from build123d import *

# Parameters (mm, degrees)
SKETCH1_W               = 202.2
SKETCH1_H               = 40
SKETCH1_R               = 1.65
BOSS_EXTRUDE1_DEPTH     = 4
SKETCH2_W               = 162.2
SKETCH2_H               = 40
CUT_EXTRUDE1_DEPTH      = 4
BOSS_EXTRUDE3_DEPTH     = 40
CUT_EXTRUDE2_DEPTH      = 184.624181414
CUT_EXTRUDE2_DEPTH_BACK = 184.624181414
SKETCH4_R               = 1.5
CUT_EXTRUDE3_DEPTH      = 104.644633243
CUT_EXTRUDE3_DEPTH_BACK = 104.644633243
SKETCH5_R               = 1.5


with BuildPart() as part:
    # Sketch1 → Boss-Extrude1 (new body)
    with BuildSketch(Plane.XY):
        Rectangle(SKETCH1_W, SKETCH1_H)
        with Locations((-95.1, 10)):
            Circle(SKETCH1_R, mode=Mode.SUBTRACT)
        with Locations((-95.1, -10)):
            Circle(SKETCH1_R, mode=Mode.SUBTRACT)
        with Locations(Location((95.1, -10, 0), (0, 0, 180))):
            Circle(SKETCH1_R, mode=Mode.SUBTRACT)
        with Locations(Location((95.1, 10, 0), (0, 0, 180))):
            Circle(SKETCH1_R, mode=Mode.SUBTRACT)
    extrude(amount=BOSS_EXTRUDE1_DEPTH)

    # Sketch2 → Cut-Extrude1 (cut)
    with BuildSketch(Plane.XY.offset(4)):
        Rectangle(SKETCH2_W, SKETCH2_H)
    extrude(amount=-CUT_EXTRUDE1_DEPTH, mode=Mode.SUBTRACT)


with BuildPart() as cut_extrude1_piece_1:
    # of the separate pieces the step leaves, piece 1, a body of its own (cut_extrude1_pieces)
    add(part.part.solids().sort_by_distance((-101.1, 20, 0))[0])



with BuildPart() as cut_extrude1_piece_2:
    # of the separate pieces the step leaves, piece 2, a body of its own (cut_extrude1_pieces)
    add(part.part.solids().sort_by_distance((81.1, 20, 0))[0])


with BuildPart() as cut_extrude1_piece_1_1:
    add(cut_extrude1_piece_1.part)

    add(cut_extrude1_piece_2.part)  # Boss-Extrude3 merges Cut-Extrude1 piece 2
    # Sketch3 → Boss-Extrude3 (add)
    with BuildSketch(Plane.XZ.offset(20)):
        Polygon((-81.1, 4), (-77.1, 4), (-77.1, -7), (77.1, -7), (77.1, 4), (81.1, 4), (81.1, -11), (-81.1, -11), align=None)
    extrude(amount=-BOSS_EXTRUDE3_DEPTH)

    # Sketch4 → Cut-Extrude2 (cut, two sides: drawn at the far end of the back side and taken through both)
    with BuildSketch(Plane.ZY.offset(81.1).offset(-CUT_EXTRUDE2_DEPTH_BACK)):
        with Locations((-4, 10)):
            Circle(SKETCH4_R)
        with Locations((-4, -10)):
            Circle(SKETCH4_R)
    extrude(amount=CUT_EXTRUDE2_DEPTH + CUT_EXTRUDE2_DEPTH_BACK, mode=Mode.SUBTRACT)

    # Sketch5 → Cut-Extrude3 (cut, two sides: drawn at the far end of the back side and taken through both)
    with BuildSketch(Plane.XY.offset(-7).offset(-CUT_EXTRUDE3_DEPTH_BACK)):
        with Locations((-11.665, 11.665)):
            Circle(SKETCH5_R)
        with Locations((11.665, 11.665)):
            Circle(SKETCH5_R)
        with Locations((11.665, -11.665)):
            Circle(SKETCH5_R)
        with Locations((-11.665, -11.665)):
            Circle(SKETCH5_R)
    extrude(amount=CUT_EXTRUDE3_DEPTH + CUT_EXTRUDE3_DEPTH_BACK, mode=Mode.SUBTRACT)


solid = cut_extrude1_piece_1_1.part
Could you check a few things on this model? Use its own coordinates, in mm. A direction names the side the tool comes from. Give positions to 0.01 mm unless a question says otherwise; leave off trailing zeros. Order: outer loops, then holes, each group sorted by start corner. A loop starts at its lowest first (then second) coordinate and runs counter-clockwise, first axis right, second up. Notation, with made-up numbers: (7.25, 75) - (40.25, 75) arc R29 cw to (40.25, 104) - close; hole circle Ø4 at (57, -11.75). An arc over 180 degrees is marked (long way). Return JSON: item names as keys, results as strings. Group by question number.
Q1. Suppose I cut it at B-B, the plane z = -9.25. Please give me the cut outline in (x, y) (3 decimals).
Q2. Please list where these lines run through material, in increasing order: line 1 along Y through (x, z) = (-95.1, 3.15); line 2 along Y through (x, z) = (79.5, -4); line 3 along X through (y, z) = (10.5, -0.75). Write a range as [from, to].
Q3. Will these pins go through, and if not, where does the flat tip stop? pin 1 Ø3.5 at (x, y) = (11.665, 11.665) entering from -Z; pin 2 Ø5.5 at (y, z) = (5, -3) entering from +X; pin 3 Ø3.5 at (y, z) = (5, -4.5) entering from -X; pin 4 Ø12 at (x, y) = (10, -9) entering from +Z.
Q4. Which directions (+Z, -Z, +X, -X, +Y, -Y) give clear straight access to the entire face, cutting with the end or side of a thin tool? Please do faces 4 (the face through (-81.1, 0, -6)), 5 (the face through (91, 0, 0)), 6 (the face through (77.1, 0, -2)).
Q5. Thinking about a two-plate mould opening in X: for faces 1 (the face through (81.1, 0, -5)), 2 (the face through (-1, 0, -7)), 3 (the face through (-89, 0, 4)), which applies, pulls with the +X half, pulls with the -X half, needs draft (parallel to the pull), parting line crosses it, or undercut?
Q6. Suppose I cut it at A-A, the plane y = 16.5. Please give me the cut outline in (x, z), and give its area (3 significant figures).
Q7. Suppose I cut it at C-C, the plane x = -72. Please give me the cut outline in (y, z), and give its area (3 significant figures).
Resolved:
{
 "1": {"outline": "(-81.1, -20) - (81.1, -20) - (81.1, 20) - (-81.1, 20) - close; hole circle Ø3 at (-11.665, -11.665); hole circle Ø3 at (-11.665, 11.665); hole circle Ø3 at (11.665, -11.665); hole circle Ø3 at (11.665, 11.665)"},
 "2": {"line 1": "y = [-20, -11.65], [-8.35, 8.35], [11.65, 20]", "line 2": "y = [-20, -11.5], [-8.5, 8.5], [11.5, 20]", "line 3": "x = [-81.1, -77.1], [77.1, 81.1]"},
 "3": {"pin 1": "stops at z = -11", "pin 2": "stops at x = 81.1", "pin 3": "stops at x = -81.1", "pin 4": "stops at z = -7"},
 "4": {"face 4": "-Z, -X, +Y, -Y", "face 5": "-Z, +X, +Y, -Y", "face 6": "+Z, +Y, -Y"},
 "5": {"face 1": "pulls with the +X half", "face 2": "undercut", "face 3": "needs draft"},
 "6": {"outline": "(-101.1, 0) - (-81.1, 0) - (-81.1, -11) - (81.1, -11) - (81.1, 0) - (101.1, 0) - (101.1, 4) - (77.1, 4) - (77.1, -7) - (-77.1, -7) - (-77.1, 4) - (-101.1, 4) - close", "area": "897 mm2"},
 "7": {"outline": "(-20, -11) - (20, -11) - (20, -7) - (-20, -7) - close", "area": "160 mm2"}
}
